Geometry: see drawing. Coordinates: mm, zero at the bounding-box minimum. A direction names the side the tool comes from. Round coordinates to 2 decimals unless told otherwise and drop trailing zeros. Order: outer loops, then holes, each group sorted by start corner. A loop starts at its lowest first (then second) coordinate and runs counter-clockwise, first axis right, second up. Notation, with made-up numbers: (81.25, 37) -> (128.25, 37) arc R26 cw to (128.25, 73) -> close; hole circle Ø10 at (61.25, 25.5). An arc over 180 degrees is marked (long way). Answer as CSV lines item,"result". Start each with the question number.
(1) Section query B-B (y = 12.7). Output: boundary loops of the cut face in (x, z) (1 decimal).
(2) Section query C-C (x = 12.7). Output: boundary loops of the cut face in (y, z) (1 decimal), plus the area to 3 significant figures.
(3) Set-up query: the marked faces 1 and 2. Return all of +Z, -Z, +X, -X, +Y, -Y with unobstructed straight access to the full face (end or side cutting, diameter ignored); none if empty.
(4) Contact query for flat-ended pins moving along their axis: P1, Ø1, axis at y = 22, z = 28, coming from the -X side; P2, Ø3, axis at y = 12.7, z = 38.1, coming from the +X side; P3, Ø1.5, axis at y = 30, z = 16.5, coming from the +X side (3 decimals); P4, Ø5.5, axis at x = 12.7, y = 12.7, coming from the -Z side (3 decimals). Output: stop coordinate, or through.
(5) Section query A-A (z = 12.7). Output: boundary loops of the cut face in (x, y) (1 decimal).
(6) Section query D-D (y = 6). Output: boundary loops of the cut face in (x, z) (1 decimal), plus the area to 3 significant figures.
(7) Line query: line 1 along Y through (x, z) = (0.85, 38.1); line 2 along Z through (x, y) = (10, 30) (1 decimal); line 3 along X through (y, z) = (46, 11.5) (1 decimal). Output: solid intervals per line, ascending. Write a range as from..to.
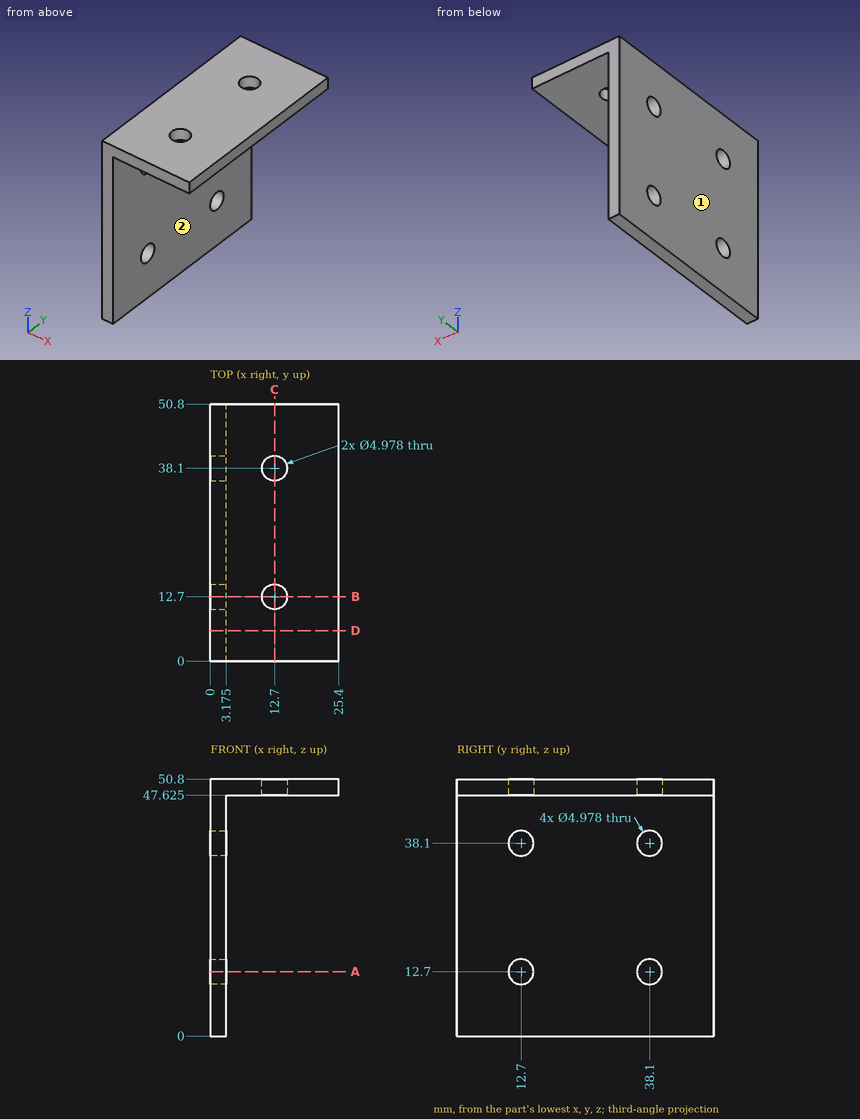
Answer block:
1,outline,"(0, 0) -> (3.2, 0) -> (3.2, 10.2) -> (0, 10.2) -> close; (0, 15.2) -> (3.2, 15.2) -> (3.2, 35.6) -> (0, 35.6) -> close; (0, 40.6) -> (3.2, 40.6) -> (3.2, 47.6) -> (10.2, 47.6) -> (10.2, 50.8) -> (0, 50.8) -> close; (15.2, 47.6) -> (25.4, 47.6) -> (25.4, 50.8) -> (15.2, 50.8) -> close"
2,outline,"(0, 47.6) -> (10.2, 47.6) -> (10.2, 50.8) -> (0, 50.8) -> close; (15.2, 47.6) -> (35.6, 47.6) -> (35.6, 50.8) -> (15.2, 50.8) -> close; (40.6, 47.6) -> (50.8, 47.6) -> (50.8, 50.8) -> (40.6, 50.8) -> close"
2,area,"130 mm2"
3,face 1,"+Z, -Z, -X, +Y, -Y"
3,face 2,"-Z, +X, +Y, -Y"
4,P1,"x = 0"
4,P2,"through"
4,P3,"x = 3.175"
4,P4,"z = 47.625"
5,outline,"(0, 0) -> (3.2, 0) -> (3.2, 10.2) -> (0, 10.2) -> close; (0, 15.2) -> (3.2, 15.2) -> (3.2, 35.6) -> (0, 35.6) -> close; (0, 40.6) -> (3.2, 40.6) -> (3.2, 50.8) -> (0, 50.8) -> close"
6,outline,"(0, 0) -> (3.2, 0) -> (3.2, 47.6) -> (25.4, 47.6) -> (25.4, 50.8) -> (0, 50.8) -> close"
6,area,"232 mm2"
7,line 1,"0..10.21, 15.19..35.61, 40.59..50.8"
7,line 2,"47.6..50.8"
7,line 3,"0..3.2"
